from build123d import *

# Parameters (mm, degrees)
F0_R     = 8.73125
F1_DEPTH = 12.7
F2_R     = 8.73125
F3_DEPTH = 30.1625
F5_DEPTH = 17.4625
F7_DEPTH = 9.525
F9_DEPTH = 12.7


with BuildPart() as f1:
    # F0 (on Top) → F1 (new body)
    with BuildSketch(Plane.XY):
        with BuildLine():
            ThreePointArc((-88.9, -7.9375), (-81.460512, -25.898012), (-63.5, -33.3375))
            ThreePointArc((-63.5, -33.3375), (-45.539488, -25.898012), (-38.1, -7.9375))
            ThreePointArc((-38.1, -7.9375), (-63.5, 17.4625), (-88.9, -7.9375))
        make_face()
        with Locations((-63.5, -7.9375)):
            Circle(F0_R, mode=Mode.SUBTRACT)
        with BuildLine():
            ThreePointArc((-38.1, -7.9375), (-45.539488, -25.898012), (-63.5, -33.3375))
            Line((-63.5, -33.3375), (63.5, -33.3375))
            ThreePointArc((63.5, -33.3375), (45.539488, 10.023012), (88.9, -7.9375))
            Line((88.9, -7.9375), (88.9, 33.3375))
            Line((88.9, 33.3375), (-88.9, 33.3375))
            Line((-88.9, 33.3375), (-88.9, -7.9375))
            ThreePointArc((-88.9, -7.9375), (-63.5, 17.4625), (-38.1, -7.9375))
        make_face()
        with BuildLine():
            ThreePointArc((88.9, -7.9375), (45.539488, 10.023012), (63.5, -33.3375))
            ThreePointArc((63.5, -33.3375), (81.460512, -25.898012), (88.9, -7.9375))
        make_face()
        with Locations((63.5, -7.9375)):
            Circle(F0_R, mode=Mode.SUBTRACT)
    extrude(amount=F1_DEPTH)

    # F2 (on Right) → F3 (join, symmetric)
    with BuildSketch(Plane.YZ):
        with BuildLine():
            Line((-33.3375, 63.5), (-33.3375, 12.7))
            Line((-33.3375, 12.7), (-7.9375, 12.7))
            Line((-7.9375, 12.7), (33.3375, 12.7))
            Line((33.3375, 12.7), (33.3375, 73.025))
            Line((33.3375, 73.025), (20.6375, 73.025))
            Line((20.6375, 73.025), (2.849747, 83.844552))
            ThreePointArc((2.849747, 83.844552), (11.232033, 75.169651), (14.2875, 63.5))
            ThreePointArc((14.2875, 63.5), (-9.525, 39.6875), (-33.3375, 63.5))
        make_face()
        with BuildLine():
            ThreePointArc((2.849747, 83.844552), (-21.194651, 84.257033), (-33.3375, 63.5))
            ThreePointArc((-33.3375, 63.5), (-9.525, 39.6875), (14.2875, 63.5))
            ThreePointArc((14.2875, 63.5), (11.232033, 75.169651), (2.849747, 83.844552))
        make_face()
        with Locations((-9.525, 63.5)):
            Circle(F2_R, mode=Mode.SUBTRACT)
    extrude(amount=F3_DEPTH, both=True)

    # F4 (on Right) → F5 (cut, symmetric)
    with BuildSketch(Plane.YZ):
        with BuildLine():
            Line((-33.3375, 12.7), (-7.9375, 12.7))
            Line((-7.9375, 12.7), (20.6375, 12.7))
            Line((20.6375, 12.7), (20.6375, 73.025))
            Line((20.6375, 73.025), (2.849747, 83.844552))
            ThreePointArc((2.849747, 83.844552), (-21.194651, 84.257033), (-33.3375, 63.5))
            Line((-33.3375, 63.5), (-33.3375, 12.7))
        make_face()
    extrude(amount=F5_DEPTH, both=True, mode=Mode.SUBTRACT)

    # F6 (on face) → F7 (join)
    with BuildSketch(Plane.XZ.offset(33.3375)):
        Polygon((-30.1625, 31.75), (-49.2125, 12.7), (-30.1625, 12.7), align=None)
        Polygon((30.1625, 31.75), (30.1625, 12.7), (49.2125, 12.7), align=None)
    extrude(amount=-F7_DEPTH)

    # F8 (on face) → F9 (join, through all)
    with BuildSketch(Plane(origin=(0, 33.3375, 0), x_dir=(-1, 0, 0), z_dir=(0, 1, 0))):
        with BuildLine():
            ThreePointArc((-30.1625, 63.5), (-45.041476, 27.578976), (-80.9625, 12.7))
            Line((-80.9625, 12.7), (-30.1625, 12.7))
            Line((-30.1625, 12.7), (-30.1625, 63.5))
        make_face()
        with BuildLine():
            ThreePointArc((80.9625, 12.7), (45.041476, 27.578976), (30.1625, 63.5))
            Line((30.1625, 63.5), (30.1625, 12.7))
            Line((30.1625, 12.7), (80.9625, 12.7))
        make_face()
    extrude(amount=-F9_DEPTH)


solid = f1.part
Could you check a few things on this model? Use its own coordinates, in mm. A direction names the side the tool comes from. Give positions to 0.01 mm unless a question says otherwise; leave off trailing zeros. Write each loop counter-clockwise with the first axis right and the second up, starting at its lowest first coordinate (ties: lowest second). Pieces come first, ordered by that corner, then holes. Notation, with made-up numbers: (19, 5.25) -> (78, 5.25) arc R4 cw to (78, 12.25) -> close; hole circle Ø4 at (-30, -19). An arc over 180 degrees is marked (long way). Answer as CSV lines item,"result". Start each with the question number.
(1) Please list where these lines run through material, in increasing order: line 1 (X direction, y = 2.5, z = 31); line 2 (Y direction, x = -63.5, z = 4.5); line 3 (Y direction, x = -24, z = 63.5).
(2) If we section it at D-D, the plane z = 22: Write out the boundary of the cut face in (x, y).
(3) If we section it at C-C, the plane y = 17.5: Write out the boundary of the cut face in (x, z).
(4) Which directions (+Z, -Z, +X, -X, +Y, -Y) give clear straight access to the entire face, cutting with the end or side of a thin tool? Please do faces 5 (the face through (0, 27, 73.025)), 6 (the face through (23.901, -20.886, 84.428)), 7 (the face through (0, -7, 12.7)), 8 (the face through (39.82, -28.64, 22.09)), 9 (the face through (30.162, -8, 51)).
(5) If we section it at B-B, the plane x = 67.5: Write out the boundary of the cut face in (y, z), and give its area (3 significant figures).
(6) If we section it at A-A, the plane z = 82: Write out the boundary of the cut face in (x, y).
(7) I'm going to push flat-ended pins straight in: pin 1 Ø8 at (x, y) = (-61.5, -1.5) entering from +Z; pin 2 Ø8 at (x, z) = (-9, 56.5) entering from -Y; pin 3 Ø10 at (x, y) = (-9, 24.5) entering from +Z (3 decimals); pin 4 Ø15.5 at (y, z) = (-9.525, 63.5) entering from +X. Where does each tip first touch, or does it pass through?
(8) If we mould it in two halves opening along X, with no side actions, what happens to faces 1 (the face through (17.462, -7, 51)), 2 (the face through (-30.162, -8, 51)), 3 (the face through (-17.462, -7, 51)), 4 (the face through (-23.72, 11.87, 78.36))? For each: +X half, -X half, draft (parallel to the pull), parting line (faces both ways), or undercut.
Answer list:
1,line 1,"-30.16 to -17.46, 17.46 to 30.16"
1,line 2,"-33.34 to -16.67, 0.79 to 33.34"
1,line 3,"-33.34 to -18.26, -0.79 to 33.34"
2,outline,"(-51.66, 20.64) -> (-30.16, 20.64) -> (-30.16, -23.81) -> (-39.91, -23.81) -> (-39.91, -33.34) -> (-17.46, -33.34) -> (-17.46, 20.64) -> (17.46, 20.64) -> (17.46, -33.34) -> (39.91, -33.34) -> (39.91, -23.81) -> (30.16, -23.81) -> (30.16, 20.64) -> (51.66, 20.64) -> (51.66, 33.34) -> (-51.66, 33.34) -> close"
3,outline,"(-88.9, 0) -> (88.9, 0) -> (88.9, 12.7) -> (30.16, 12.7) -> (30.16, 74.93) -> (17.46, 74.93) -> (17.46, 12.7) -> (-17.46, 12.7) -> (-17.46, 74.93) -> (-30.16, 74.93) -> (-30.16, 12.7) -> (-88.9, 12.7) -> close"
4,face 5,"+Z, +X, -X, +Y"
4,face 6,"+Z, +X, -X"
4,face 7,"+Z, -Y"
4,face 8,"+Z, +X, -Y"
4,face 9,"+Z, +X"
5,outline,"(-33.02, 0) -> (-15.7, 0) -> (-15.7, 12.7) -> (-33.02, 12.7) -> close; (-0.18, 0) -> (33.34, 0) -> (33.34, 14.52) -> (20.64, 14.52) -> (20.64, 12.7) -> (-0.18, 12.7) -> close"
5,area,"669 mm^2"
6,outline,"(-30.16, -24.52) -> (-17.46, -24.52) -> (-17.46, 5.88) -> (-30.16, 5.88) -> close; (17.46, -24.52) -> (30.16, -24.52) -> (30.16, 5.88) -> (17.46, 5.88) -> close"
7,pin 1,"z = 12.7"
7,pin 2,"y = 20.64"
7,pin 3,"z = 73.025"
7,pin 4,"through"
8,face 1,"undercut"
8,face 2,"-X half"
8,face 3,"undercut"
8,face 4,"draft"
